from build123d import *

# Parameters (mm, degrees)
EXTRUDE_1_DEPTH     = 2
SKETCH_2_R          = 1.05
SKETCH_2_R_2        = 1.05760355
CUT_EXTRUDE_1_DEPTH = 6
CUT_EXTRUDE_2_DEPTH = 4


with BuildPart() as part:
    # 草图1 → 凸台-拉伸1 (new body)
    with BuildSketch(Plane.XY):
        Polygon((-4.597711938, -13.43249055), (-4.597711938, -38.43249055), (-29.597711938, -38.43249055), (-29.597711938, -40.43249055), (-34.597711938, -40.43249055), (-39.597711938, -40.43249055), (-39.597711938, -38.43249055), (-64.597711938, -38.43249055), (-64.597711938, -13.43249055), (-66.597711938, -13.43249055), (-66.597711938, -8.43249055), (-66.597711938, -3.43249055), (-64.597711938, -3.43249055), (-64.597711938, 21.56750945), (-39.597711938, 21.56750945), (-39.597711938, 23.56750945), (-29.597711938, 23.56750945), (-29.597711938, 21.56750945), (-4.597711938, 21.56750945), (-4.597711938, -3.43249055), (-2.597711938, -3.43249055), (-2.597711938, -13.43249055), align=None)
    extrude(amount=EXTRUDE_1_DEPTH)

    # 草图2 → 切除-拉伸1 (cut)
    with BuildSketch(Plane.XY):
        with Locations(Location((-50.075826656, 17.046317073, 0), (0, 0, 180))):
            Circle(SKETCH_2_R)
        with Locations(Location((-19.146292681, 17.004293118, 0), (0, 0, 180))):
            Circle(SKETCH_2_R_2)
        with Locations(Location((-19.146292681, -33.910264006, 0), (0, 0, 180))):
            Circle(SKETCH_2_R)
        with Locations(Location((-50.075826656, -33.910264006, 0), (0, 0, 180))):
            Circle(SKETCH_2_R)
    extrude(amount=CUT_EXTRUDE_1_DEPTH, mode=Mode.SUBTRACT)

    # 草图4 → 切除-拉伸2 (cut)
    with BuildSketch(Plane.XY):
        Polygon((-32.878676175, 18.720597517), (-22.611059668, 18.720597517), (-22.611059668, 15.325305096), (-32.878676175, 15.325305096), (-46.611059668, 15.325305096), (-46.611059668, 18.720597517), align=None)
    extrude(amount=CUT_EXTRUDE_2_DEPTH, mode=Mode.SUBTRACT)


solid = part.part
The listing builds one solid part. Answer for the finished solid, in the listing's coordinates (mm). A direction names the side the tool comes from. Coordinates: 2 decimals unless noted, no trailing zeros. Write each loop counter-clockwise with the first axis right and the second up, starting at its lowest first coordinate (ties: lowest second). Pieces come first, ordered by that corner, then holes. Notation, with made-up numbers: M 20,46.25 L 33,46.25 A8 cw 33,50.25 Z; hole C 23.5,36.5 d10. An arc over 180 degrees is marked long. Use one line per item in the form item = value.
Item 1: For faces 1 (the face through (-52, -38.432, 1)), 2 (the face through (-29.598, 23, 1)), 3 (the face through (-66, -3.432, 1)), determine the directions among +Z, -Z, +X, -X, +Y, -Y from which every point of the face is accessible in a straight line to the end or side of a thin tool.
Model answer:
face_1 = +Z, -Z, -X, -Y
face_2 = +Z, -Z, +X, +Y
face_3 = +Z, -Z, -X, +Y
Item 2: Find section C-C, the plane x = -42.5. Give the vertices of the cut face in (y, z), plus the area to 3 significant figures.
Model answer:
outline = M -38.43,0 L 15.33,0 L 15.33,2 L -38.43,2 Z; M 18.72,0 L 21.57,0 L 21.57,2 L 18.72,2 Z
area = 113 mm2
Item 3: Find section B-B, the plane z = 1.35. Give the vertices of the cut face in (x, y).
Model answer:
outline = M -66.6,-13.43 L -64.6,-13.43 L -64.6,-38.43 L -39.6,-38.43 L -39.6,-40.43 L -29.6,-40.43 L -29.6,-38.43 L -4.6,-38.43 L -4.6,-13.43 L -2.6,-13.43 L -2.6,-3.43 L -4.6,-3.43 L -4.6,21.57 L -29.6,21.57 L -29.6,23.57 L -39.6,23.57 L -39.6,21.57 L -64.6,21.57 L -64.6,-3.43 L -66.6,-3.43 Z; hole C -50.08,-33.91 d2.1; hole C -50.08,17.05 d2.1; hole M -46.61,15.33 L -22.61,15.33 L -22.61,18.72 L -46.61,18.72 Z; hole C -19.15,-33.91 d2.1; hole C -19.15,17 d2.12
Item 4: Find the intervals of material crossed by probe 1 along X at (y, z) = (17, 1.05); probe 2 along Y at (x, z) = (-28, 1); probe 3 along Y at (x, z) = (-36, 1.9), in increasing order.
Model answer:
probe_1 = -64.6 to -51.12, -49.03 to -46.61, -22.61 to -20.2, -18.09 to -4.6
probe_2 = -38.43 to 15.33, 18.72 to 21.57
probe_3 = -40.43 to 15.33, 18.72 to 23.57
Item 5: Find section A-A, the plane x = -31.5. Give the vertices of the cut face in (y, z), plus the area to 3 significant figures.
Model answer:
outline = M -40.43,0 L 15.33,0 L 15.33,2 L -40.43,2 Z; M 18.72,0 L 23.57,0 L 23.57,2 L 18.72,2 Z
area = 121 mm2
Item 6: Given P1, Ø0.6, axis at y = 23, z = 0.5, coming from the -X side; P2, Ø0.6, axis at x = -16, z = 1, coming from the -Y side; P3, Ø0.6, axis at y = -39.5, z = 1, coming from the +X side, each flat-ended and moving along its own axis, determine where each tip first touches the part or whether it passes through.
Model answer:
P1 = -39.6
P2 = -38.43
P3 = -29.6
Item 7: Find section D-D, the plane y = 12.5. Give the vertices of the cut face in (x, z).
Model answer:
outline = M -64.6,0 L -4.6,0 L -4.6,2 L -64.6,2 Z
Item 8: The mould has two halves that part along Y. Classify faces 4 (the face through (-34, 18.721, 1)), 5 (the face through (-17, 21.568, 1)), 6 (the face through (-34, -8, 0)): released by +Y, released by -Y, zero draft, split by the parting line, or undercut.
Model answer:
face_4 = undercut
face_5 = released by +Y
face_6 = zero draft
